```python
from build123d import *

# Parameters (mm, degrees)
SKETCH1_W                 = 255.3
SKETCH1_H                 = 94.3
BOSS_EXTRUDE1_DEPTH       = 4
ADVANCEDHOLE2_OUTLINE_R   = 2.25
ADVANCEDHOLE2_DEPTH       = 2.23
ADVANCEDHOLE2_DRAFT       = -45
ADVANCEDHOLE2_2_OUTLINE_R = 2.25
ADVANCEDHOLE2_2_DEPTH     = 2.23
ADVANCEDHOLE2_2_DRAFT     = -45
ADVANCEDHOLE2_3_OUTLINE_R = 2.25
ADVANCEDHOLE2_3_DEPTH     = 2.23
ADVANCEDHOLE2_3_DRAFT     = -45
ADVANCEDHOLE2_4_OUTLINE_R = 2.25
ADVANCEDHOLE2_4_DEPTH     = 2.23
ADVANCEDHOLE2_4_DRAFT     = -45
ADVANCEDHOLE2_5_OUTLINE_R = 2.25
ADVANCEDHOLE2_5_DEPTH     = 2.23
ADVANCEDHOLE2_5_DRAFT     = -45
ADVANCEDHOLE2_6_OUTLINE_R = 2.25
ADVANCEDHOLE2_6_DEPTH     = 2.23
ADVANCEDHOLE2_6_DRAFT     = -45
ADVANCEDHOLE2_7_OUTLINE_R = 2.25
ADVANCEDHOLE2_7_DEPTH     = 2.23
ADVANCEDHOLE2_7_DRAFT     = -45
ADVANCEDHOLE2_8_OUTLINE_R = 2.25
ADVANCEDHOLE2_8_DEPTH     = 2.23
ADVANCEDHOLE2_8_DRAFT     = -45


# Read off the part's stored shape, not the designer's step: AdvancedHole2
with BuildPart() as part:
    # Sketch1 → Boss-Extrude1 (new body)
    with BuildSketch(Plane(origin=(0, 0, 0), x_dir=(1, 0, 0), z_dir=(0, 1, 0))):
        with Locations((127.65, 47.15)):
            Rectangle(SKETCH1_W, SKETCH1_H)
    extrude(amount=BOSS_EXTRUDE1_DEPTH)


with BuildPart() as advancedhole2_tool:
    # AdvancedHole2 outline → AdvancedHole2 (with draft: the straight prism first)
    with BuildSketch(Plane(origin=(0, 1.77, 0), x_dir=(1, 0, 0), z_dir=(0, 1, 0))):
        with Locations((231.15, 24.15)):
            Circle(ADVANCEDHOLE2_OUTLINE_R)
    extrude(amount=ADVANCEDHOLE2_DEPTH)
    # AdvancedHole2: the draft: its side faces are tilted about the plane it starts from
    advancedhole2_sides = [advancedhole2_tool.faces().sort_by_distance(p)[0] for p in [
        (228.9, 2.885, -24.15),
    ]]
    draft(advancedhole2_sides, Plane(origin=(0, 1.77, 0), x_dir=(1, 0, 0), z_dir=(0, 1, 0)), ADVANCEDHOLE2_DRAFT)


with BuildPart() as part_1:
    add(part.part)

    # AdvancedHole2: cut by advancedhole2_tool
    add(advancedhole2_tool.part, mode=Mode.SUBTRACT)


with BuildPart() as advancedhole2_2_tool:
    # AdvancedHole2 2 outline → AdvancedHole2 2 (with draft: the straight prism first)
    with BuildSketch(Plane(origin=(0, 1.77, 0), x_dir=(1, 0, 0), z_dir=(0, 1, 0))):
        with Locations((231.15, 70.15)):
            Circle(ADVANCEDHOLE2_2_OUTLINE_R)
    extrude(amount=ADVANCEDHOLE2_2_DEPTH)
    # AdvancedHole2 2: the draft: its side faces are tilted about the plane it starts from
    advancedhole2_2_sides = [advancedhole2_2_tool.faces().sort_by_distance(p)[0] for p in [
        (228.9, 2.885, -70.15),
    ]]
    draft(advancedhole2_2_sides, Plane(origin=(0, 1.77, 0), x_dir=(1, 0, 0), z_dir=(0, 1, 0)), ADVANCEDHOLE2_2_DRAFT)


with BuildPart() as part_2:
    add(part_1.part)

    # AdvancedHole2 2: cut by advancedhole2_2_tool
    add(advancedhole2_2_tool.part, mode=Mode.SUBTRACT)


with BuildPart() as advancedhole2_3_tool:
    # AdvancedHole2 3 outline → AdvancedHole2 3 (with draft: the straight prism first)
    with BuildSketch(Plane(origin=(0, 1.77, 0), x_dir=(1, 0, 0), z_dir=(0, 1, 0))):
        with Locations((162.15, 70.15)):
            Circle(ADVANCEDHOLE2_3_OUTLINE_R)
    extrude(amount=ADVANCEDHOLE2_3_DEPTH)
    # AdvancedHole2 3: the draft: its side faces are tilted about the plane it starts from
    advancedhole2_3_sides = [advancedhole2_3_tool.faces().sort_by_distance(p)[0] for p in [
        (159.9, 2.885, -70.15),
    ]]
    draft(advancedhole2_3_sides, Plane(origin=(0, 1.77, 0), x_dir=(1, 0, 0), z_dir=(0, 1, 0)), ADVANCEDHOLE2_3_DRAFT)


with BuildPart() as part_3:
    add(part_2.part)

    # AdvancedHole2 3: cut by advancedhole2_3_tool
    add(advancedhole2_3_tool.part, mode=Mode.SUBTRACT)


with BuildPart() as advancedhole2_4_tool:
    # AdvancedHole2 4 outline → AdvancedHole2 4 (with draft: the straight prism first)
    with BuildSketch(Plane(origin=(0, 1.77, 0), x_dir=(1, 0, 0), z_dir=(0, 1, 0))):
        with Locations((162.15, 24.15)):
            Circle(ADVANCEDHOLE2_4_OUTLINE_R)
    extrude(amount=ADVANCEDHOLE2_4_DEPTH)
    # AdvancedHole2 4: the draft: its side faces are tilted about the plane it starts from
    advancedhole2_4_sides = [advancedhole2_4_tool.faces().sort_by_distance(p)[0] for p in [
        (159.9, 2.885, -24.15),
    ]]
    draft(advancedhole2_4_sides, Plane(origin=(0, 1.77, 0), x_dir=(1, 0, 0), z_dir=(0, 1, 0)), ADVANCEDHOLE2_4_DRAFT)


with BuildPart() as part_4:
    add(part_3.part)

    # AdvancedHole2 4: cut by advancedhole2_4_tool
    add(advancedhole2_4_tool.part, mode=Mode.SUBTRACT)


with BuildPart() as advancedhole2_5_tool:
    # AdvancedHole2 5 outline → AdvancedHole2 5 (with draft: the straight prism first)
    with BuildSketch(Plane(origin=(0, 1.77, 0), x_dir=(1, 0, 0), z_dir=(0, 1, 0))):
        with Locations((93.15, 24.15)):
            Circle(ADVANCEDHOLE2_5_OUTLINE_R)
    extrude(amount=ADVANCEDHOLE2_5_DEPTH)
    # AdvancedHole2 5: the draft: its side faces are tilted about the plane it starts from
    advancedhole2_5_sides = [advancedhole2_5_tool.faces().sort_by_distance(p)[0] for p in [
        (90.9, 2.885, -24.15),
    ]]
    draft(advancedhole2_5_sides, Plane(origin=(0, 1.77, 0), x_dir=(1, 0, 0), z_dir=(0, 1, 0)), ADVANCEDHOLE2_5_DRAFT)


with BuildPart() as part_5:
    add(part_4.part)

    # AdvancedHole2 5: cut by advancedhole2_5_tool
    add(advancedhole2_5_tool.part, mode=Mode.SUBTRACT)


with BuildPart() as advancedhole2_6_tool:
    # AdvancedHole2 6 outline → AdvancedHole2 6 (with draft: the straight prism first)
    with BuildSketch(Plane(origin=(0, 1.77, 0), x_dir=(1, 0, 0), z_dir=(0, 1, 0))):
        with Locations((93.15, 70.15)):
            Circle(ADVANCEDHOLE2_6_OUTLINE_R)
    extrude(amount=ADVANCEDHOLE2_6_DEPTH)
    # AdvancedHole2 6: the draft: its side faces are tilted about the plane it starts from
    advancedhole2_6_sides = [advancedhole2_6_tool.faces().sort_by_distance(p)[0] for p in [
        (90.9, 2.885, -70.15),
    ]]
    draft(advancedhole2_6_sides, Plane(origin=(0, 1.77, 0), x_dir=(1, 0, 0), z_dir=(0, 1, 0)), ADVANCEDHOLE2_6_DRAFT)


with BuildPart() as part_6:
    add(part_5.part)

    # AdvancedHole2 6: cut by advancedhole2_6_tool
    add(advancedhole2_6_tool.part, mode=Mode.SUBTRACT)


with BuildPart() as advancedhole2_7_tool:
    # AdvancedHole2 7 outline → AdvancedHole2 7 (with draft: the straight prism first)
    with BuildSketch(Plane(origin=(0, 1.77, 0), x_dir=(1, 0, 0), z_dir=(0, 1, 0))):
        with Locations((24.15, 24.15)):
            Circle(ADVANCEDHOLE2_7_OUTLINE_R)
    extrude(amount=ADVANCEDHOLE2_7_DEPTH)
    # AdvancedHole2 7: the draft: its side faces are tilted about the plane it starts from
    advancedhole2_7_sides = [advancedhole2_7_tool.faces().sort_by_distance(p)[0] for p in [
        (21.9, 2.885, -24.15),
    ]]
    draft(advancedhole2_7_sides, Plane(origin=(0, 1.77, 0), x_dir=(1, 0, 0), z_dir=(0, 1, 0)), ADVANCEDHOLE2_7_DRAFT)


with BuildPart() as part_7:
    add(part_6.part)

    # AdvancedHole2 7: cut by advancedhole2_7_tool
    add(advancedhole2_7_tool.part, mode=Mode.SUBTRACT)


with BuildPart() as advancedhole2_8_tool:
    # AdvancedHole2 8 outline → AdvancedHole2 8 (with draft: the straight prism first)
    with BuildSketch(Plane(origin=(0, 1.77, 0), x_dir=(1, 0, 0), z_dir=(0, 1, 0))):
        with Locations((24.15, 70.15)):
            Circle(ADVANCEDHOLE2_8_OUTLINE_R)
    extrude(amount=ADVANCEDHOLE2_8_DEPTH)
    # AdvancedHole2 8: the draft: its side faces are tilted about the plane it starts from
    advancedhole2_8_sides = [advancedhole2_8_tool.faces().sort_by_distance(p)[0] for p in [
        (21.9, 2.885, -70.15),
    ]]
    draft(advancedhole2_8_sides, Plane(origin=(0, 1.77, 0), x_dir=(1, 0, 0), z_dir=(0, 1, 0)), ADVANCEDHOLE2_8_DRAFT)


with BuildPart() as part_8:
    add(part_7.part)

    # AdvancedHole2 8: cut by advancedhole2_8_tool
    add(advancedhole2_8_tool.part, mode=Mode.SUBTRACT)


solid = part_8.part
```
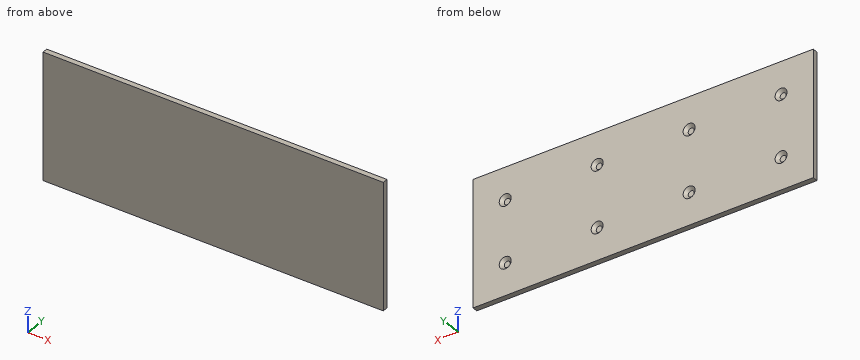
Check sheet for the modelled part. Datum: model origin and axes. Units: mm. Coordinates: 2 decimals unless noted, no trailing zeros. Loops run counter-clockwise (first coordinate to the right, second up) from the corner with the lowest first, then second, coordinate; pieces in that order, holes last.
1) Sectioned sample at B-B (x = 231.15). Record the boundary of the cut face in (y, z), and give its area (3 significant figures).
2) Material ranges on probe 1 along X at (y, z) = (2.4, -69.5), recorded low to high.
3) Gauge pin test, flat ends, axial feed: pin 1 (5 mm diameter, centred on x = 93.5, z = -71, fed in from +Y); pin 2 (1.3 mm diameter, centred on x = 231.5, z = -70.5, fed in from +Y); pin 3 (3.5 mm diameter, centred on x = 93.5, z = -25, fed in from +Y). Record the tip position at first contact, or that the pin passes through.
4) Sectioned sample at A-A (z = -70.15). Record the boundary of the cut face in (x, y).
Check sheet entries:
1. outline: (0, -94.3) - (4, -94.3) - (4, -74.63) - (1.77, -72.4) - (1.77, -67.9) - (4, -65.67) - (4, -28.63) - (1.77, -26.4) - (1.77, -21.9) - (4, -19.67) - (4, 0) - (0, 0) - close
1. area: 347 mm2
2. probe 1: x = 0 to 21.34, 26.96 to 90.34, 95.96 to 159.34, 164.96 to 228.34, 233.96 to 255.3
3. pin 1: stops at y = 2.94
3. pin 2: stops at y = 1.77
3. pin 3: stops at y = 2.19
4. outline: (0, 0) - (255.3, 0) - (255.3, 4) - (235.63, 4) - (233.4, 1.77) - (228.9, 1.77) - (226.67, 4) - (166.63, 4) - (164.4, 1.77) - (159.9, 1.77) - (157.67, 4) - (97.63, 4) - (95.4, 1.77) - (90.9, 1.77) - (88.67, 4) - (28.63, 4) - (26.4, 1.77) - (21.9, 1.77) - (19.67, 4) - (0, 4) - close
